Can you work these out from the model? Positions are in its coordinate system, mm. Face numbers are marked on the shaded views. A direction names the side the tool comes from. Coordinates: 2 decimals unless noted, no trailing zeros. Loops run counter-clockwise (first coordinate to the right, second up) from the corner with the lowest first, then second, coordinate; pieces in that order, holes last. Notation, with made-up numbers: (69, 17) - (122, 17) arc R16 ccw to (122, 42) - close; hole circle Ø9 at (-6.5, 80.5). An arc over 180 degrees is marked (long way). Put each result on its own line as item: value. Start each with the question number.
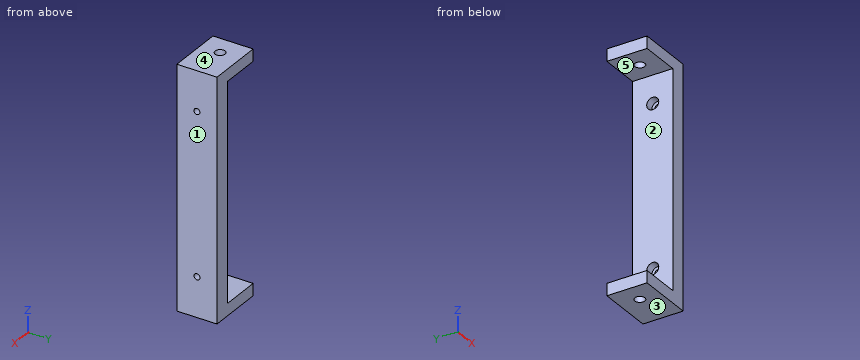
from build123d import *

# Parameters (mm, degrees)
PAD003_DEPTH        = 10
HOLE004_D           = 3
HOLE004_DEPTH       = 25
HOLE004_CBORE_D     = 6
HOLE004_CBORE_DEPTH = 4
SKETCH009_R         = 2.5
POCKET_DEPTH        = 6.001
POCKET_DEPTH_BACK   = 113.501


with BuildPart() as part:
    # Sketch007 → Pad003 (new body, symmetric)
    with BuildSketch(Plane.XZ):
        Polygon((0, 53.75), (-20, 53.75), (-20, 59.75), (8, 59.75), (8, -59.75), (-20, -59.75), (-20, -53.75), (0, -53.75), align=None)
    extrude(amount=PAD003_DEPTH, both=True)

    # Hole004
    with Locations(Plane(origin=(0, 0, 0), x_dir=(0, 0, -1), z_dir=(-1, 0, 0))):
        with Locations((-40, 0), (40, 0)):
            CounterBoreHole(HOLE004_D / 2, HOLE004_CBORE_D / 2, HOLE004_CBORE_DEPTH, depth=HOLE004_DEPTH)

    # Sketch009 (on Face1 of Hole004) → Pocket (cut, two sides)
    with BuildSketch(Plane(origin=(0, 0, 53.75), x_dir=(1, 0, 0), z_dir=(0, 0, -1))) as pocket_sk:
        with Locations((-10, 0)):
            Circle(SKETCH009_R)
    extrude(amount=-POCKET_DEPTH, mode=Mode.SUBTRACT)
    extrude(pocket_sk.sketch, amount=POCKET_DEPTH_BACK, mode=Mode.SUBTRACT)


solid = part.part
Q1. I want a section at C-C on x = -6.5. List the corners of the cut face in (y, z) for me, and give its area (3 significant figures).
Q2. I want a section at B-B on z = -40. List the corners of the cut face in (x, y) for me.
Q3. On a 3-axis mill with a long thin cutter (end or side, diameter ignored), from which of +Z, -Z, +X, -X, +Y, -Y can I reach the whole of each face in a straight line? I mean the marked faces 4 and 5. Say none if no direction works.
Q4. Will these pins go through, and if not, where does the flat tip stop? pin 1 (5 mm diameter, centred on y = 4.5, z = -20, fed in from -X); pin 2 (3 mm diameter, centred on y = 0, z = 39, fed in from -X); pin 3 (4.5 mm diameter, centred on x = -10, y = 0, fed in from -Z); pin 4 (8 mm diameter, centred on x = -10, y = 0, fed in from +Z).
Q5. I want a section at A-A on y = 0. Count the separate pieces of the cut face and the enclosed holes in it, and give its area (3 significant figures).
Q6. I want a section at D-D on y = -6. List the corners of the cut face in (x, z) for me.
Q7. Please list where these lines run through material, in increasing order: line 1 along Z through (x, y) = (-6.75, 5.25); line 2 along Y through (x, z) = (3.25, 40); line 3 along Y through (x, z) = (-10, 58.3). Write a range as [from, to].
Q8. We'd pull the mould along Z, two halves only. Please class the marked faces 1, 2 and 3: released by +Z, released by -Z, zero draft, split by the parting line, or undercut.
Calculated:
1. outline: (-10, -59.75) - (10, -59.75) - (10, -53.75) - (-10, -53.75) - close; (-10, 53.75) - (10, 53.75) - (10, 59.75) - (-10, 59.75) - close
1. area: 240 mm2
2. outline: (0, -10) - (8, -10) - (8, -1.5) - (4, -1.5) - (4, -3) - (0, -3) - close; (0, 3) - (4, 3) - (4, 1.5) - (8, 1.5) - (8, 10) - (0, 10) - close
3. face 4: +Z, +X, -X, +Y, -Y
3. face 5: -X, +Y, -Y
4. pin 1: x = 0
4. pin 2: x = 4
4. pin 3: through
4. pin 4: z = 59.75
5. separate pieces: 5
5. enclosed holes: 0
5. area: 1,060 mm2
6. outline: (-20, -59.75) - (8, -59.75) - (8, 59.75) - (-20, 59.75) - (-20, 53.75) - (0, 53.75) - (0, -53.75) - (-20, -53.75) - close
7. line 1: [-59.75, -53.75], [53.75, 59.75]
7. line 2: [-10, -3], [3, 10]
7. line 3: [-10, -2.5], [2.5, 10]
8. face 1: zero draft
8. face 2: undercut
8. face 3: released by -Z
